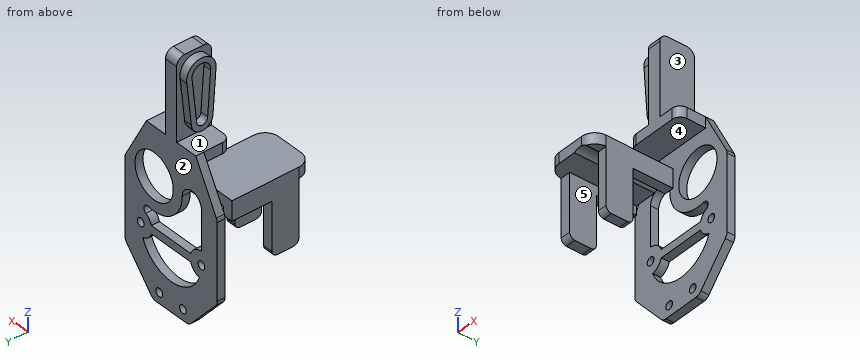
```python
from build123d import *

# Parameters (mm, degrees)
SKETCH1_R            = 1.5
SKETCH1_R_2          = 8.5
BOSS_EXTRUDE1_DEPTH  = 1.5
FILLET1_R            = 3
BOSS_EXTRUDE2_DEPTH  = 30
SKETCH7_W            = 3.75
SKETCH7_H            = 23.325864092
BOSS_EXTRUDE4_DEPTH  = 25
SKETCH10_W           = 3.45
SKETCH10_H           = 25
BOSS_EXTRUDE15_DEPTH = 23
SKETCH11_W           = 3.75
SKETCH11_H           = 15
CUT_EXTRUDE1_DEPTH   = 20
SKETCH12_W           = 3.45
SKETCH12_H           = 15
CUT_EXTRUDE2_DEPTH   = 20
SKETCH13_W           = 22
SKETCH13_H           = 4
BOSS_EXTRUDE16_DEPTH = 10
SKETCH14_W           = 2.5
SKETCH14_H           = 13
BOSS_EXTRUDE17_DEPTH = 30
FILLET3_R            = 3
FILLET4_R            = 3
FILLET5_R            = 3
FILLET6_R            = 3
FILLET7_R            = 2
FILLET8_R            = 2
FILLET9_R            = 2
FILLET10_R           = 2
FILLET11_R           = 5
FILLET12_R           = 5
BOSS_EXTRUDE18_DEPTH = 3


with BuildPart() as part:
    # Sketch1 → Boss-Extrude1 (new body, symmetric)
    with BuildSketch(Plane(origin=(0, 0, 0), x_dir=(1, 0, 0), z_dir=(0, 1, 0))):
        Polygon((8, 24.400284093), (-8, 24.400284093), (-20.5, 10), (-20.5, -20), (-11, -37.599715907), (11, -37.599715907), (20.5, -20), (20.5, 10), align=None)
        with Locations((-5.25, 20.39454584)):
            Circle(SKETCH1_R, mode=Mode.SUBTRACT)
        with Locations((5.25, 20.39454584)):
            Circle(SKETCH1_R, mode=Mode.SUBTRACT)
        with Locations((-13.5, 0)):
            Circle(SKETCH1_R, mode=Mode.SUBTRACT)
        with Locations((13.5, 0)):
            Circle(SKETCH1_R, mode=Mode.SUBTRACT)
        with Locations((7.530163354, -19.817414772)):
            Circle(SKETCH1_R_2, mode=Mode.SUBTRACT)
        with BuildLine():
            Line((-13.5, -5), (-13.5, -19.817414772))
            ThreePointArc((-13.5, -19.817414772), (-9.234918323, -24.082496449), (-4.969836646, -19.817414772))
            ThreePointArc((-4.969836646, -19.817414772), (-0.361028795, -10.12313365), (10.06681719, -7.57750516))
            ThreePointArc((10.06681719, -7.57750516), (11.99598649, -6.493442694), (11.187975781, -4.433344563))
            ThreePointArc((11.187975781, -4.433344563), (9.667400631, -3.211102938), (8.730303993, -1.5))
            Line((8.730303993, -1.5), (-8.730303993, -1.5))
            ThreePointArc((-8.730303993, -1.5), (-10.541960108, -4.031128874), (-13.5, -5))
        make_face(mode=Mode.SUBTRACT)
        with BuildLine():
            Line((8.730303993, 1.5), (-8.730303993, 1.5))
            ThreePointArc((-8.730303993, 1.5), (-10.179901517, 3.738575405), (-12.574074074, 4.913518208))
            ThreePointArc((-12.574074074, 4.913518208), (0, 13.5), (12.574074074, 4.913518208))
            ThreePointArc((12.574074074, 4.913518208), (10.179901517, 3.738575405), (8.730303993, 1.5))
        make_face(mode=Mode.SUBTRACT)
    extrude(amount=BOSS_EXTRUDE1_DEPTH, both=True)

    # Fillet1
    fillet1_edges = [part.edges().sort_by_distance(p)[0] for p in [
        (-20.5, 0, 20),
        (-20.5, 0, -10),
        (-8, 0, -24.400284093),
        (8, 0, -24.400284093),
        (20.5, 0, -10),
        (20.5, 0, 20),
    ]]
    fillet(fillet1_edges, radius=FILLET1_R)

    # Sketch4 → Boss-Extrude2 (add)
    with BuildSketch(Plane.XZ.offset(1.5)):
        Polygon((-23.5, 27.325864092), (-23.5, 23.325864092), (-18.70476029, 23.325864092), (-16.545634529, 27.325864092), align=None)
        with BuildLine():
            Line((-18.70476029, 23.325864092), (-13.5, 23.325864092))
            Line((-13.5, 23.325864092), (-11.660141009, 23.325864092))
            ThreePointArc((-11.660141009, 23.325864092), (-9.234918323, 24.082496449), (-6.809695637, 23.325864092))
            Line((-6.809695637, 23.325864092), (-3.5, 23.325864092))
            Line((-3.5, 23.325864092), (-3.5, 27.325864092))
            Line((-3.5, 27.325864092), (-16.545634529, 27.325864092))
            Line((-16.545634529, 27.325864092), (-18.70476029, 23.325864092))
        make_face()
    extrude(amount=BOSS_EXTRUDE2_DEPTH)

    # Sketch7 → Boss-Extrude4 (add)
    with BuildSketch(Plane.XZ.offset(1.5)):
        with Locations((-21.625, 11.662932046)):
            Rectangle(SKETCH7_W, SKETCH7_H)
    extrude(amount=BOSS_EXTRUDE4_DEPTH)

    # Sketch10 → Boss-Extrude15 (add)
    with BuildSketch(Plane(origin=(0, 0, 23.325864092), x_dir=(-1, 0, 0), z_dir=(0, 0, -1))):
        with Locations((5.225, -14)):
            Rectangle(SKETCH10_W, SKETCH10_H)
    extrude(amount=BOSS_EXTRUDE15_DEPTH)

    # Sketch11 → Cut-Extrude1 (cut)
    with BuildSketch(Plane(origin=(0, 0, 0), x_dir=(-1, 0, 0), z_dir=(0, 0, -1))):
        with Locations((21.625, -9)):
            Rectangle(SKETCH11_W, SKETCH11_H)
    extrude(amount=-CUT_EXTRUDE1_DEPTH, mode=Mode.SUBTRACT)

    # Sketch12 → Cut-Extrude2 (cut)
    with BuildSketch(Plane(origin=(0, 0, 0.325864092), x_dir=(-1, 0, 0), z_dir=(0, 0, -1))):
        with Locations((5.225, -9)):
            Rectangle(SKETCH12_W, SKETCH12_H)
    extrude(amount=-CUT_EXTRUDE2_DEPTH, mode=Mode.SUBTRACT)

    # Sketch13 → Boss-Extrude16 (add)
    with BuildSketch(Plane.XZ.offset(1.5)):
        with Locations((0, 35.599715907)):
            Rectangle(SKETCH13_W, SKETCH13_H)
    extrude(amount=BOSS_EXTRUDE16_DEPTH)

    # Sketch14 → Boss-Extrude17 (add)
    with BuildSketch(Plane.XY.offset(37.599715907)):
        with Locations((1.25, -5)):
            Rectangle(SKETCH14_W, SKETCH14_H)
        with Locations((-1.25, -5)):
            Rectangle(SKETCH14_W, SKETCH14_H)
    extrude(amount=BOSS_EXTRUDE17_DEPTH)

    # Fillet3
    fillet3_edges = [part.edges().sort_by_distance(p)[0] for p in [
        (-11, -11.5, 35.599715907),
    ]]
    fillet(fillet3_edges, radius=FILLET3_R)

    # Fillet4
    fillet4_edges = [part.edges().sort_by_distance(p)[0] for p in [
        (11, -11.5, 35.599715907),
    ]]
    fillet(fillet4_edges, radius=FILLET4_R)

    # Fillet5
    fillet5_edges = [part.edges().sort_by_distance(p)[0] for p in [
        (0, 1.5, 67.599715907),
    ]]
    fillet(fillet5_edges, radius=FILLET5_R)

    # Fillet6
    fillet6_edges = [part.edges().sort_by_distance(p)[0] for p in [
        (0, -11.5, 67.599715907),
    ]]
    fillet(fillet6_edges, radius=FILLET6_R)

    # Fillet7
    fillet7_edges = [part.edges().sort_by_distance(p)[0] for p in [
        (-21.625, -16.5, 0),
    ]]
    fillet(fillet7_edges, radius=FILLET7_R)

    # Fillet8
    fillet8_edges = [part.edges().sort_by_distance(p)[0] for p in [
        (-21.625, -26.5, 0),
    ]]
    fillet(fillet8_edges, radius=FILLET8_R)

    # Fillet9
    fillet9_edges = [part.edges().sort_by_distance(p)[0] for p in [
        (-5.225, -26.5, 0.325864092),
    ]]
    fillet(fillet9_edges, radius=FILLET9_R)

    # Fillet10
    fillet10_edges = [part.edges().sort_by_distance(p)[0] for p in [
        (-5.225, -16.5, 0.325864092),
    ]]
    fillet(fillet10_edges, radius=FILLET10_R)

    # Fillet11
    fillet11_edges = [part.edges().sort_by_distance(p)[0] for p in [
        (-3.5, -31.5, 25.325864092),
    ]]
    fillet(fillet11_edges, radius=FILLET11_R)

    # Fillet12
    fillet12_edges = [part.edges().sort_by_distance(p)[0] for p in [
        (-23.5, -31.5, 25.325864092),
    ]]
    fillet(fillet12_edges, radius=FILLET12_R)

    # Sketch15 → Boss-Extrude18 (add)
    with BuildSketch(Plane.ZY.offset(2.5)):
        with BuildLine():
            Line((60.019494917, -10.664595798), (44.083601773, -9.563551575))
            ThreePointArc((44.083601773, -9.563551575), (40.114289707, -5.53663584), (44.039052889, -1.466289101))
            Line((44.039052889, -1.466289101), (59.646971548, 0.211283454))
            ThreePointArc((59.646971548, 0.211283454), (66.207952811, -5.008307663), (60.019494917, -10.664595798))
        make_face()
        with BuildLine():
            Line((60.218460063, -8.673574683), (44.164228414, -7.564354205))
            ThreePointArc((44.164228414, -7.564354205), (42.114228414, -5.514354205), (44.164228414, -3.464354205))
            Line((44.164228414, -3.464354205), (59.955274566, -1.767098714))
            ThreePointArc((59.955274566, -1.767098714), (64.208636435, -5.063268193), (60.218460063, -8.673574683))
        make_face(mode=Mode.SUBTRACT)
    extrude(amount=BOSS_EXTRUDE18_DEPTH)


solid = part.part
```
Input: part model. Units: mm. Frame: model coordinates. Face numbers are marked on the shaded views. A direction names the side the tool comes from. Coordinates: 2 decimals unless noted, no trailing zeros. Write each loop counter-clockwise with the first axis right and the second up, starting at its lowest first coordinate (ties: lowest second). Pieces come first, ordered by that corner, then holes. Notation, with made-up numbers: (32, 30) - (67, 30) arc R7 ccw to (67, 40) - close; hole circle Ø1 at (-26.5, 25). An arc over 180 degrees is marked (long way). Put each result on its own line as item: value. Start each with the question number.
1) Cut plane B-B (x = 13.5). Return the cut outline in (y, z).
2) Ray query, L1, parallel to Z at x = 5.25, y = 0.2; L2, parallel to Z at x = 10, y = 0; L3, parallel to Z at x = 13.5, y = -0.2. Return the intervals inside material, ascending.
3) Reachability of the marked faces 3, 4 and 5 from +Z, -Z, +X, -X, +Y, -Y: full face, straight path, thin tool, end or side. Return the list, or none.
4) Cut plane A-A (y = -14.5). Return the cut outline in (x, z), plus the area to 3 significant figures.
5) Mould query, pull axis Z, two halves, no side actions, for the marked faces 1 and 2. Classes: pulls with the +Z half, pulls with the -Z half, needs draft (parallel to the pull), parting line crosses it, or undercut.
6) Cut plane D-D (z = 53). Return the cut outline in (x, y).
7) Cut plane C-C (x = 5.25). Return the cut outline in (y, z).
8) Contact query for flat-ended pins moving along their axis: pin 1 (2.5 mm diameter, centred on x = -13.5, z = 0, fed in from +Y); pin 2 (1.7 mm diameter, centred on x = -6, y = -12.5, fed in from -Z); pin 3 (5.5 mm diameter, centred on y = -6, z = 51.5, fed in from -X); pin 4 (9.5 mm diameter, centred on x = 8, y = -3, fed in from +Z). Output: stop coordinate, or through.
Resolved:
1. outline: (-1.5, -18.06) - (1.5, -18.06) - (1.5, -1.5) - (-1.5, -1.5) - close; (-1.5, 1.5) - (1.5, 1.5) - (1.5, 13.77) - (-1.5, 13.77) - close; (-1.5, 25.87) - (1.5, 25.87) - (1.5, 32.97) - (-1.5, 32.97) - close
2. L1: z = -24.4 to -21.89, -18.89 to -12.44, -1.5 to 1.5, 7.53 to 11.63, 28.01 to 37.6
2. L2: z = -22.1 to -9.07, -3.57 to 3.57, 7.56 to 11.68, 27.95 to 37.6
2. L3: z = -18.06 to -1.5, 1.5 to 13.77, 25.87 to 32.97
3. face 3: +Z, +X, +Y, -Y
3. face 4: +X, -X, -Y
3. face 5: -Z, -Y
4. outline: (-23.5, 20) - (-19.75, 20) - (-19.75, 23.33) - (-11.66, 23.33) arc R4.27 cw to (-6.81, 23.33) - (-6.95, 23.33) - (-6.95, 20.33) - (-3.5, 20.33) - (-3.5, 27.33) - (-23.5, 27.33) - close
4. area: 100 mm2
5. face 1: undercut
5. face 2: needs draft
6. outline: (-5.5, -10.18) - (-2.5, -10.18) - (-2.5, -11.5) - (2.5, -11.5) - (2.5, 1.5) - (-2.5, 1.5) - (-2.5, -0.5) - (-5.5, -0.5) - (-5.5, -2.51) - (-2.5, -2.51) - (-2.5, -8.17) - (-5.5, -8.17) - close
7. outline: (-11.5, 33.6) - (-1.5, 33.6) - (-1.5, 28.01) - (1.5, 28.01) - (1.5, 37.6) - (-11.5, 37.6) - close; (-1.5, -24.4) - (1.5, -24.4) - (1.5, -21.89) - (-1.5, -21.89) - close; (-1.5, -18.89) - (1.5, -18.89) - (1.5, -12.44) - (-1.5, -12.44) - close; (-1.5, -1.5) - (1.5, -1.5) - (1.5, 1.5) - (-1.5, 1.5) - close; (-1.5, 7.53) - (1.5, 7.53) - (1.5, 11.63) - (-1.5, 11.63) - close
8. pin 1: passes through
8. pin 2: stops at z = 20.33
8. pin 3: stops at x = -5.5
8. pin 4: stops at z = 37.6
